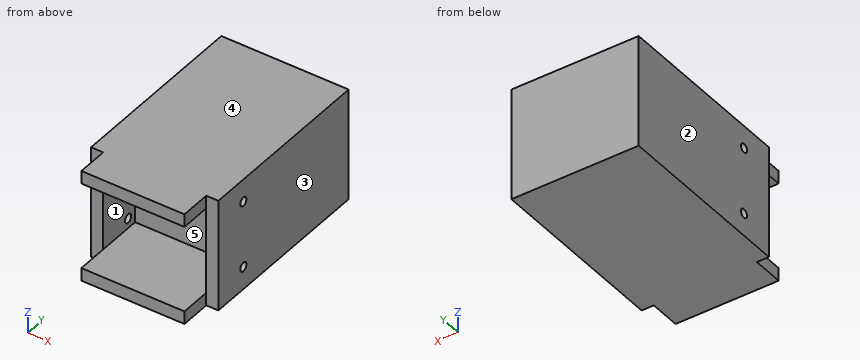
```python
from build123d import *

# Parameters (mm, degrees)
SKETCH1_W               = 50
SKETCH1_H               = 150
BOSS_EXTRUDE1_DEPTH     = 55
CUT_EXTRUDE1_DEPTH      = 168.406690428
CUT_EXTRUDE1_DEPTH_BACK = 45
SKETCH2_R               = 10.25
SKETCH7_R               = 1
SKETCH7_R_2             = 4.25
CUT_EXTRUDE3_DEPTH      = 10
SKETCH8_W               = 55
SKETCH8_H               = 55
SKETCH8_R               = 10.25
BOSS_EXTRUDE2_DEPTH     = 50
SKETCH10_W              = 8
SKETCH10_H              = 10.25
SKETCH10_W_2            = 17
SKETCH10_H_2            = 1
SKETCH10_W_3            = 34
SKETCH10_H_3            = 20
SKETCH10_H_4            = 5
CUT_EXTRUDE4_DEPTH      = 214.717102732
SKETCH11_W              = 34
SKETCH11_H              = 13.25
BOSS_EXTRUDE4_DEPTH     = 25
SKETCH13_W              = 55
SKETCH13_H              = 10
CUT_EXTRUDE5_DEPTH      = 8
SKETCH14_R              = 5.030159043
CUT_EXTRUDE6_DEPTH      = 8
SKETCH15_W              = 34
SKETCH15_H              = 0.25
BOSS_EXTRUDE5_DEPTH     = 13.25
CUT_EXTRUDE7_DEPTH      = 181.416185527
BOSS_EXTRUDE6_START     = 1.5
SKETCH19_R              = 10.25
SKETCH19_R_2            = 1
SKETCH19_R_3            = 4.25
BOSS_EXTRUDE6_DEPTH     = 1.5
CUT_EXTRUDE8_DEPTH      = 184.89467094
SKETCH21_R              = 5.030159043
SKETCH21_R_2            = 4.5
BOSS_EXTRUDE7_DEPTH     = 8
SKETCH24_W              = 4
SKETCH24_H              = 30
CUT_EXTRUDE10_DEPTH     = 181.416185527
SKETCH25_W              = 55
SKETCH25_H              = 86.25
CUT_EXTRUDE11_DEPTH     = 4
BOSS_EXTRUDE8_START     = 4
SKETCH26_R              = 1
SKETCH26_R_2            = 4.25
BOSS_EXTRUDE8_DEPTH     = 4
SKETCH27_W              = 4
SKETCH27_H              = 123.25
CUT_EXTRUDE12_DEPTH     = 181.416185527
CUT_EXTRUDE13_DEPTH     = 180.905530765
SKETCH29_W              = 42
SKETCH29_H              = 9
CUT_EXTRUDE15_DEPTH     = 174.776436838
SKETCH30_R              = 4.5
SKETCH30_R_2            = 1.45
BOSS_EXTRUDE9_DEPTH     = 4
SKETCH31_W              = 37
SKETCH31_H              = 55
CUT_EXTRUDE16_DEPTH     = 182.05247858
SKETCH32_W              = 93.338891709
SKETCH32_H              = 62.145945894
CUT_EXTRUDE17_DEPTH     = 182.05247858


with BuildPart() as part:
    # Sketch1 → Boss-Extrude1 (new body)
    with BuildSketch(Plane.XY):
        with Locations((0, -75)):
            Rectangle(SKETCH1_W, SKETCH1_H)
    extrude(amount=-BOSS_EXTRUDE1_DEPTH)

    # Sketch2 → Cut-Extrude1 (cut, two sides: drawn at the far end of the back side and taken through both)
    with BuildSketch(Plane(origin=(25, 0, 0), x_dir=(0, 0, -1), z_dir=(1, 0, 0)).offset(-CUT_EXTRUDE1_DEPTH_BACK)):
        with Locations(Location((27.5, -25, 0), (0, 0, 270))):
            Circle(SKETCH2_R)
    extrude(amount=CUT_EXTRUDE1_DEPTH + CUT_EXTRUDE1_DEPTH_BACK, mode=Mode.SUBTRACT)

    # Sketch7 → Cut-Extrude3 (cut)
    with BuildSketch(Plane(origin=(-20, 0, 0), x_dir=(0, 0, -1), z_dir=(1, 0, 0))):
        with Locations(Location((27.5, -17, 0), (0, 0, 90))):
            Circle(SKETCH7_R)
        with Locations(Location((35.5, -25, 0), (0, 0, 90))):
            Circle(SKETCH7_R)
        with Locations(Location((27.5, -33, 0), (0, 0, 90))):
            Circle(SKETCH7_R)
        with Locations(Location((19.5, -25, 0), (0, 0, 90))):
            Circle(SKETCH7_R)
        with Locations(Location((27.5, -25, 0), (0, 0, 90))):
            Circle(SKETCH7_R_2)
    extrude(amount=-CUT_EXTRUDE3_DEPTH, mode=Mode.SUBTRACT)

    # Sketch8 → Boss-Extrude2 (add)
    with BuildSketch(Plane(origin=(25, 0, 0), x_dir=(0, 0, -1), z_dir=(1, 0, 0))):
        with Locations((27.5, -177.5)):
            Rectangle(SKETCH8_W, SKETCH8_H)
        with Locations(Location((27.5, -180, 0), (0, 0, 90))):
            Circle(SKETCH8_R, mode=Mode.SUBTRACT)
    extrude(amount=-BOSS_EXTRUDE2_DEPTH)

    # Sketch10 → Cut-Extrude4 (cut, through all)
    with BuildSketch(Plane.XY):
        Polygon((-17, -205), (17, -205), (17, -191.25), (0, -191.25), (-17, -191.25), align=None)
        Polygon((-25, -205), (-17, -205), (-17, -191.25), (-17, -190.25), (-25, -190.25), align=None)
        Polygon((17, -191.25), (17, -205), (25, -205), (25, -190.25), (17, -190.25), align=None)
        with Locations((-21, -185.125)):
            Rectangle(SKETCH10_W, SKETCH10_H)
        with Locations((-21, -174.875)):
            Rectangle(SKETCH10_W, SKETCH10_H)
        with Locations((21, -174.875)):
            Rectangle(SKETCH10_W, SKETCH10_H)
        with Locations((21, -185.125)):
            Rectangle(SKETCH10_W, SKETCH10_H)
        with Locations((-8.5, -185.125)):
            Rectangle(SKETCH10_W_2, SKETCH10_H)
        with Locations((8.5, -185.125)):
            Rectangle(SKETCH10_W_2, SKETCH10_H)
        Polygon((0, -180), (17, -180), (17, -169.75), (-17, -169.75), (-17, -180), align=None)
        with Locations((-8.5, -190.75)):
            Rectangle(SKETCH10_W_2, SKETCH10_H_2)
        with Locations((8.5, -190.75)):
            Rectangle(SKETCH10_W_2, SKETCH10_H_2)
        with Locations((0, -154.75)):
            Rectangle(SKETCH10_W_3, SKETCH10_H_3)
        with Locations((0, -167.25)):
            Rectangle(SKETCH10_W_3, SKETCH10_H_4)
    extrude(amount=-CUT_EXTRUDE4_DEPTH, mode=Mode.SUBTRACT)

    # Sketch11 → Boss-Extrude4 (add)
    with BuildSketch(Plane.XZ.offset(144.75)):
        with Locations((0, -6.625)):
            Rectangle(SKETCH11_W, SKETCH11_H)
        with Locations((0, -48.375)):
            Rectangle(SKETCH11_W, SKETCH11_H)
    extrude(amount=BOSS_EXTRUDE4_DEPTH)

    # Sketch13 → Cut-Extrude5 (cut)
    with BuildSketch(Plane(origin=(25, 0, 0), x_dir=(0, 0, -1), z_dir=(1, 0, 0))):
        with Locations((27.5, -164.75)):
            Rectangle(SKETCH13_W, SKETCH13_H)
    cut_extrude5 = extrude(amount=-CUT_EXTRUDE5_DEPTH, mode=Mode.SUBTRACT)

    # Mirror2: Cut-Extrude5 across plane
    add(cut_extrude5.mirror(Plane(origin=(0, 0, 0), x_dir=(0, 0, 1), z_dir=(1, 0, 0))), mode=Mode.SUBTRACT)

    # Sketch14 → Cut-Extrude6 (cut)
    with BuildSketch(Plane(origin=(25, 0, 0), x_dir=(0, 0, -1), z_dir=(1, 0, 0))):
        with Locations(Location((16.5, -148, 0), (0, 0, 90))):
            Circle(SKETCH14_R)
        with Locations(Location((38.5, -148, 0), (0, 0, 90))):
            Circle(SKETCH14_R)
    cut_extrude6 = extrude(amount=-CUT_EXTRUDE6_DEPTH, mode=Mode.SUBTRACT)

    # Mirror3: Cut-Extrude6 across plane
    add(cut_extrude6.mirror(Plane(origin=(0, 0, 0), x_dir=(0, 0, 1), z_dir=(1, 0, 0))), mode=Mode.SUBTRACT)

    # Sketch15 → Boss-Extrude5 (add)
    with BuildSketch(Plane.XY):
        with Locations((0, -169.875)):
            Rectangle(SKETCH15_W, SKETCH15_H)
    boss_extrude5 = extrude(amount=-BOSS_EXTRUDE5_DEPTH)

    # Mirror4: Boss-Extrude5 across plane
    add(boss_extrude5.mirror(Plane.XY.offset(-27.5)))

    # Sketch16 → Cut-Extrude7 (cut, through all)
    with BuildSketch(Plane.XY):
        Polygon((-18.5, 0), (-18.5, -14.75), (-18.5, -35.25), (-18.5, -43.5), (25, -43.5), (25, 0), align=None)
    extrude(amount=-CUT_EXTRUDE7_DEPTH, mode=Mode.SUBTRACT)

    # Sketch19 → Boss-Extrude6 (add)
    with BuildSketch(Plane(origin=(-20, 0, 0), x_dir=(0, 0, -1), z_dir=(1, 0, 0)).offset(BOSS_EXTRUDE6_START)):
        with Locations((27.5, -25)):
            Circle(SKETCH19_R)
        with Locations(Location((27.5, -17, 0), (0, 0, 90))):
            Circle(SKETCH19_R_2, mode=Mode.SUBTRACT)
        with Locations(Location((27.5, -33, 0), (0, 0, 90))):
            Circle(SKETCH19_R_2, mode=Mode.SUBTRACT)
        with Locations(Location((19.5, -25, 0), (0, 0, 90))):
            Circle(SKETCH19_R_2, mode=Mode.SUBTRACT)
        with Locations(Location((35.5, -25, 0), (0, 0, 90))):
            Circle(SKETCH19_R_2, mode=Mode.SUBTRACT)
        with Locations(Location((27.5, -25, 0), (0, 0, 90))):
            Circle(SKETCH19_R_3, mode=Mode.SUBTRACT)
    extrude(amount=-BOSS_EXTRUDE6_DEPTH)

    # Sketch20 → Cut-Extrude8 (cut, through all)
    with BuildSketch(Plane(origin=(-18.5, 0, 0), x_dir=(0, 0, -1), z_dir=(1, 0, 0))):
        with BuildLine():
            Line((0, 0), (0, -43.5))
            Line((0, -43.5), (9, -43.5))
            Line((9, -43.5), (9, -25))
            ThreePointArc((9, -25), (27.5, -6.5), (46, -25))
            Line((46, -25), (46, -43.5))
            Line((46, -43.5), (55, -43.5))
            Line((55, -43.5), (55, 0))
            Line((55, 0), (0, 0))
        make_face()
    extrude(amount=-CUT_EXTRUDE8_DEPTH, mode=Mode.SUBTRACT)

    # Sketch21 → Boss-Extrude7 (add)
    # profile 1 of 2: a face of its own
    with BuildSketch(Plane(origin=(25, 0, 0), x_dir=(0, 0, -1), z_dir=(1, 0, 0))):
        with Locations(Location((16.5, -148, 0), (0, 0, 229.751587581))):
            Circle(SKETCH21_R)
        with Locations(Location((16.5, -148, 0), (0, 0, 90))):
            Circle(SKETCH21_R_2, mode=Mode.SUBTRACT)
    # profile 2 of 2: a face of its own
    with BuildSketch(Plane(origin=(25, 0, 0), x_dir=(0, 0, -1), z_dir=(1, 0, 0))):
        with Locations(Location((38.5, -148, 0), (0, 0, 310.248412419))):
            Circle(SKETCH21_R)
        with Locations(Location((38.5, -148, 0), (0, 0, 90))):
            Circle(SKETCH21_R_2, mode=Mode.SUBTRACT)
    boss_extrude7 = extrude(amount=-BOSS_EXTRUDE7_DEPTH)

    # Mirror5: Boss-Extrude7 across plane
    add(boss_extrude7.mirror(Plane(origin=(0, 0, 0), x_dir=(0, 0, 1), z_dir=(1, 0, 0))))

    # Sketch24 → Cut-Extrude10 (cut, through all)
    with BuildSketch(Plane.XY):
        with Locations((-23, -144.75)):
            Rectangle(SKETCH24_W, SKETCH24_H)
        with Locations((23, -144.75)):
            Rectangle(SKETCH24_W, SKETCH24_H)
    extrude(amount=-CUT_EXTRUDE10_DEPTH, mode=Mode.SUBTRACT)

    # Sketch25 → Cut-Extrude11 (cut)
    with BuildSketch(Plane(origin=(25, 0, 0), x_dir=(0, 0, -1), z_dir=(1, 0, 0))):
        with Locations((27.5, -86.625)):
            Rectangle(SKETCH25_W, SKETCH25_H)
    extrude(amount=-CUT_EXTRUDE11_DEPTH, mode=Mode.SUBTRACT)

    # Sketch26 → Boss-Extrude8 (add)
    with BuildSketch(Plane(origin=(-18.5, 0, 0), x_dir=(0, 0, -1), z_dir=(1, 0, 0)).offset(BOSS_EXTRUDE8_START)):
        with BuildLine():
            Line((46, -43.5), (46, -25))
            ThreePointArc((46, -25), (27.5, -6.5), (9, -25))
            Line((9, -25), (9, -43.5))
            Line((9, -43.5), (46, -43.5))
        make_face()
        with Locations(Location((35.5, -25, 0), (0, 0, 90))):
            Circle(SKETCH26_R, mode=Mode.SUBTRACT)
        with Locations(Location((27.5, -25, 0), (0, 0, 90))):
            Circle(SKETCH26_R_2, mode=Mode.SUBTRACT)
        with Locations(Location((19.5, -25, 0), (0, 0, 90))):
            Circle(SKETCH26_R, mode=Mode.SUBTRACT)
        with Locations(Location((27.5, -33, 0), (0, 0, 90))):
            Circle(SKETCH26_R, mode=Mode.SUBTRACT)
        with Locations(Location((27.5, -17, 0), (0, 0, 90))):
            Circle(SKETCH26_R, mode=Mode.SUBTRACT)
    extrude(amount=-BOSS_EXTRUDE8_DEPTH)

    # Sketch27 → Cut-Extrude12 (cut, through all)
    with BuildSketch(Plane.XY):
        with Locations((-23, -68.125)):
            Rectangle(SKETCH27_W, SKETCH27_H)
    extrude(amount=-CUT_EXTRUDE12_DEPTH, mode=Mode.SUBTRACT)

    # Sketch28 → Cut-Extrude13 (cut, through all)
    with BuildSketch(Plane.XY):
        with BuildLine():
            Line((21, -43.5), (-14.5, -43.5))
            ThreePointArc((-14.5, -43.5), (10.602290732, -53.897709268), (21, -79))
            Line((21, -79), (21, -43.5))
        make_face()
    extrude(amount=-CUT_EXTRUDE13_DEPTH, mode=Mode.SUBTRACT)

    # Sketch29 → Cut-Extrude15 (cut, through all)
    with BuildSketch(Plane.XZ.offset(170)):
        with Locations((0, -50.5)):
            Rectangle(SKETCH29_W, SKETCH29_H)
        with Locations((0, -4.5)):
            Rectangle(SKETCH29_W, SKETCH29_H)
    extrude(amount=-CUT_EXTRUDE15_DEPTH, mode=Mode.SUBTRACT)

    # Sketch30 → Boss-Extrude9 (add)
    # profile 1 of 2: a face of its own
    with BuildSketch(Plane(origin=(21, 0, 0), x_dir=(0, 0, -1), z_dir=(1, 0, 0))):
        with Locations(Location((16.5, -148, 0), (0, 0, 223.761742693))):
            Circle(SKETCH30_R)
        with Locations((16.5, -148)):
            Circle(SKETCH30_R_2, mode=Mode.SUBTRACT)
    # profile 2 of 2: a face of its own
    with BuildSketch(Plane(origin=(21, 0, 0), x_dir=(0, 0, -1), z_dir=(1, 0, 0))):
        with Locations(Location((38.5, -148, 0), (0, 0, 316.238257307))):
            Circle(SKETCH30_R)
        with Locations((38.5, -148)):
            Circle(SKETCH30_R_2, mode=Mode.SUBTRACT)
    boss_extrude9 = extrude(amount=-BOSS_EXTRUDE9_DEPTH)

    # Mirror6: Boss-Extrude9 across plane
    add(boss_extrude9.mirror(Plane(origin=(0, 0, 0), x_dir=(0, 0, 1), z_dir=(1, 0, 0))))

    # Sketch31 → Cut-Extrude16 (cut, through all)
    with BuildSketch(Plane.ZY.offset(21)):
        with Locations((-27.5, -71)):
            Rectangle(SKETCH31_W, SKETCH31_H)
    extrude(amount=-CUT_EXTRUDE16_DEPTH, mode=Mode.SUBTRACT)


with BuildPart() as cut_extrude16_piece_1:
    # of the separate pieces the step leaves, piece 1, a body of its own (cut_extrude16_pieces)
    add(part.part.solids().sort_by_distance((17, -170, -13.25))[0])


with BuildPart() as cut_extrude16_piece_2:
    # of the separate pieces the step leaves, piece 2, a body of its own (cut_extrude16_pieces)
    add(part.part.solids().sort_by_distance((-21, -43.5, -9))[0])

    # Sketch32 → Cut-Extrude17 (cut, through all)
    with BuildSketch(Plane.ZY.offset(21)):
        with Locations((-22.821058128, -34.382182034)):
            Rectangle(SKETCH32_W, SKETCH32_H)
    extrude(amount=-CUT_EXTRUDE17_DEPTH, mode=Mode.SUBTRACT)


solid = cut_extrude16_piece_1.part
```
Build history of the part. All positions in model axes, mm. Face numbers are marked on the shaded views. A direction names the side the tool comes from. Coordinates: 2 decimals unless noted, no trailing zeros. Write each loop counter-clockwise with the first axis right and the second up, starting at its lowest first coordinate (ties: lowest second). Pieces come first, ordered by that corner, then holes.
1. Pull direction X, two halves, no side cores. Call the marked faces 1, 2 and 3: released by +X, released by -X, zero draft, split by the parting line, or undercut.
Answer block:
face 1: undercut
face 2: released by -X
face 3: released by +X
2. Band-saw the part on B-B, the plane z = -16.5. Give the cut face in (x, y), and give its area (3 significant figures).
Answer block:
outline: (-21, -159.75) - (-17, -159.75) - (-17, -149.45) - (-21, -149.45) - close; (-21, -146.55) - (-17, -146.55) - (-17, -144.75) - (17, -144.75) - (17, -146.55) - (21, -146.55) - (21, -98.5) - (-21, -98.5) - close; (17, -159.75) - (21, -159.75) - (21, -149.45) - (17, -149.45) - close
area: 2,040 mm2
3. Band-saw the part on A-A, the plane y = -148. Give the cut face in (x, z), and give its area (3 significant figures).
Answer block:
outline: (-21, -46) - (21, -46) - (21, -39.95) - (17, -39.95) - (17, -41.75) - (-17, -41.75) - (-17, -39.95) - (-21, -39.95) - close; (-21, -37.05) - (-17, -37.05) - (-17, -17.95) - (-21, -17.95) - close; (-21, -15.05) - (-17, -15.05) - (-17, -13.25) - (17, -13.25) - (17, -15.05) - (21, -15.05) - (21, -9) - (-21, -9) - close; (17, -37.05) - (21, -37.05) - (21, -17.95) - (17, -17.95) - close
area: 539 mm2
4. 3-axis set-ups, long thin cutter, end or side, ignore diameter. For the marked faces 4 and 5: which of +Z, -Z, +X, -X, +Y, -Y reach the whole face in a straight line?
Answer block:
face 4: +Z, +X, -X, +Y, -Y
face 5: -Y
5. Band-saw the part on D-D, the plane x = 4. Give the cut face in (y, z), and give its area (3 significant figures).
Answer block:
outline: (-170, -46) - (-98.5, -46) - (-98.5, -9) - (-170, -9) - (-170, -13.25) - (-144.75, -13.25) - (-144.75, -41.75) - (-170, -41.75) - close
area: 1,930 mm2
6. Drop flat-ended pins along their axis: pin 1 (1.3 mm diameter, centred on y = -163.5, z = -44, fed in from -X); pin 2 (8 mm diameter, centred on x = 5, z = -30, fed in from -Y); pin 3 (4.5 mm diameter, centred on x = 19.5, z = -28.5, fed in from -Y). Give the stop position or say it passes through.
Answer block:
pin 1: stops at x = -17
pin 2: stops at y = -144.75
pin 3: stops at y = -159.75
7. Drill centre lines: probe 1 along Z at (x, y) = (19.8, -148); probe 2 along X at (y, z) = (-158, -27.5); probe 3 along Y at (x, z) = (19.8, -38.5). Where is each one in solid material? Low to high.
Answer block:
probe 1: z = -46 to -39.95, -37.05 to -17.95, -15.05 to -9
probe 2: x = -21 to -17, 17 to 21
probe 3: y = -159.75 to -149.45, -146.55 to -98.5
8. Band-saw the part on C-C, the plane y = -160.5. Give the cut face in (x, z), and give its area (3 significant figures).
Answer block:
outline: (-17, -46) - (17, -46) - (17, -41.75) - (-17, -41.75) - close; (-17, -13.25) - (17, -13.25) - (17, -9) - (-17, -9) - close
area: 289 mm2
